```python
from build123d import *

# Parameters (mm, degrees)
F0_R     = 15.926715
F1_DEPTH = 73.914


with BuildPart() as f1:
    # F0 (on Front) → F1 (new body)
    with BuildSketch(Plane.XZ):
        with BuildLine():
            Line((-32.508995, -59.810236), (32.508995, -59.810236))
            Line((32.508995, -59.810236), (32.508995, 59.810236))
            Line((32.508995, 59.810236), (32.387727, 59.810236))
            ThreePointArc((32.387727, 59.810236), (0, 92.197963), (-32.387727, 59.810236))
            Line((-32.387727, 59.810236), (-32.508995, 59.810236))
            Line((-32.508995, 59.810236), (-32.508995, -59.810236))
        make_face()
        with Locations((0, 59.810236)):
            Circle(F0_R, mode=Mode.SUBTRACT)
    extrude(amount=F1_DEPTH)


solid = f1.part
```
Input: part model. Units: mm. Frame: model coordinates. Give positions to 0.01 mm unless a question says otherwise; leave off trailing zeros. Order: outer loops, then holes, each group sorted by start corner. A loop starts at its lowest first (then second) coordinate and runs counter-clockwise, first axis right, second up. Notation, with made-up numbers: M 39.25,78 L 97.25,78 A26 cw 97.25,110 Z; hole C 41.5,87.25 d1. An arc over 180 degrees is marked long. Return JSON: item names as keys, results as strings.
Item 1: Cut plane B-B (y = -33). Return loops of the section in (x, z), then the cut area to 3 significant figures.
Solutions:
{"outline": "M -32.51,-59.81 L 32.51,-59.81 L 32.51,59.81 L 32.39,59.81 A32.39 ccw -32.39,59.81 L -32.51,59.81 Z; hole C 0,59.81 d31.85", "area": "8,630 mm^2"}
Item 2: Cut plane A-A (x = 0). Return loops of the section in (y, z).
Solutions:
{"outline": "M -73.91,-59.81 L 0,-59.81 L 0,43.88 L -73.91,43.88 Z; M -73.91,75.74 L 0,75.74 L 0,92.2 L -73.91,92.2 Z"}
Item 3: First-contact query: P1, Ø3, axis at y = -32, z = 70, coming from the +X side; P2, Ø2, axis at y = -23, z = 71, coming from the -X side; P3, Ø10, axis at x = 23, z = 2, coming from the +Y side. Flat tips, straight axial feed; report the tip coordinate or a pass-through.
Solutions:
{"P1": "x = 31.2", "P2": "x = -30.74", "P3": "y = 0"}
Item 4: Pull-direction query (X, two-part tool) for faces 1 (the flat face through (0, -36, -59.81)), 2 (the flat face through (32.509, -36, -1)), 3 (the cylindrical face through (-3.45, -36.44, 44.26)); classes: +X half, -X half, draft (parallel to the pull), parting line (faces both ways), or undercut.
Solutions:
{"face 1": "draft", "face 2": "+X half", "face 3": "undercut"}
Item 5: Ray query, probe 1 along Z at (x, y) = (0, -26.5); probe 2 along X at (y, z) = (-59, 67.5); probe 3 along Z at (x, y) = (3, -10). Return the intervals inside material, ascending.
Solutions:
{"probe 1": "-59.81 to 43.88, 75.74 to 92.2", "probe 2": "-31.46 to -13.95, 13.95 to 31.46", "probe 3": "-59.81 to 44.17, 75.45 to 92.06"}
Item 6: Cut plane C-C (z = 67). Return loops of the section in (x, y).
Solutions:
{"outline": "M -31.58,-73.91 L -14.21,-73.91 L -14.21,0 L -31.58,0 Z; M 14.21,-73.91 L 31.58,-73.91 L 31.58,0 L 14.21,0 Z"}
Item 7: Cut plane D-D (x = 22). Return loops of the section in (y, z), then the cut area to 3 significant figures.
Solutions:
{"outline": "M -73.91,-59.81 L 0,-59.81 L 0,83.58 L -73.91,83.58 Z", "area": "10,600 mm^2"}
